Drawing for the job (mm, zero at the part's lowest x, y, z). A direction names the side the tool comes from. Round coordinates to 2 decimals unless told otherwise and drop trailing zeros. Write each loop counter-clockwise with the first axis right and the second up, starting at its lowest first coordinate (ties: lowest second). Pieces come first, ordered by that corner, then holes. Notation, with made-up numbers: M -38,-31.5 L -29,-31.5 A24 ccw -29,-6.5 Z; hole C 74,2.5 d4. An arc over 180 degrees is marked long. Use a Markdown table: item, result. Add a question column.
1) Slice it at D-D on x = 4.25. Write the cut outline in (y, z), plus the area to 3 significant figures.
2) Slice it at C-C on y = 3.75. Write the cut outline in (x, z).
3) Slice it at B-B on z = 4.25. Write the cut outline in (x, y).
4) Slice it at A-A on x = 7. Write the cut outline in (y, z).
5) Wall check: probe 1 along Y at (x, z) = (5, 4.75); probe 2 along X at (y, z) = (11.5, 4.5); probe 3 along Z at (x, y) = (6.25, 12.5). Give the ranges that are in metal, low to high.
6) Drop flat-ended pins along their axis: P1, Ø2, axis at y = 17, z = 5.5, coming from the +X side; P2, Ø8, axis at x = 6.5, y = 16.5, coming from the +Z side. Give the stop position or say it passes through.
7) Which spindle directions (+Z, -Z, +X, -X, +Y, -Y) get a long thin tool onto all of the face, cutting with end or side? Do the marked faces 1, 2 and 3. Say none if no direction does.
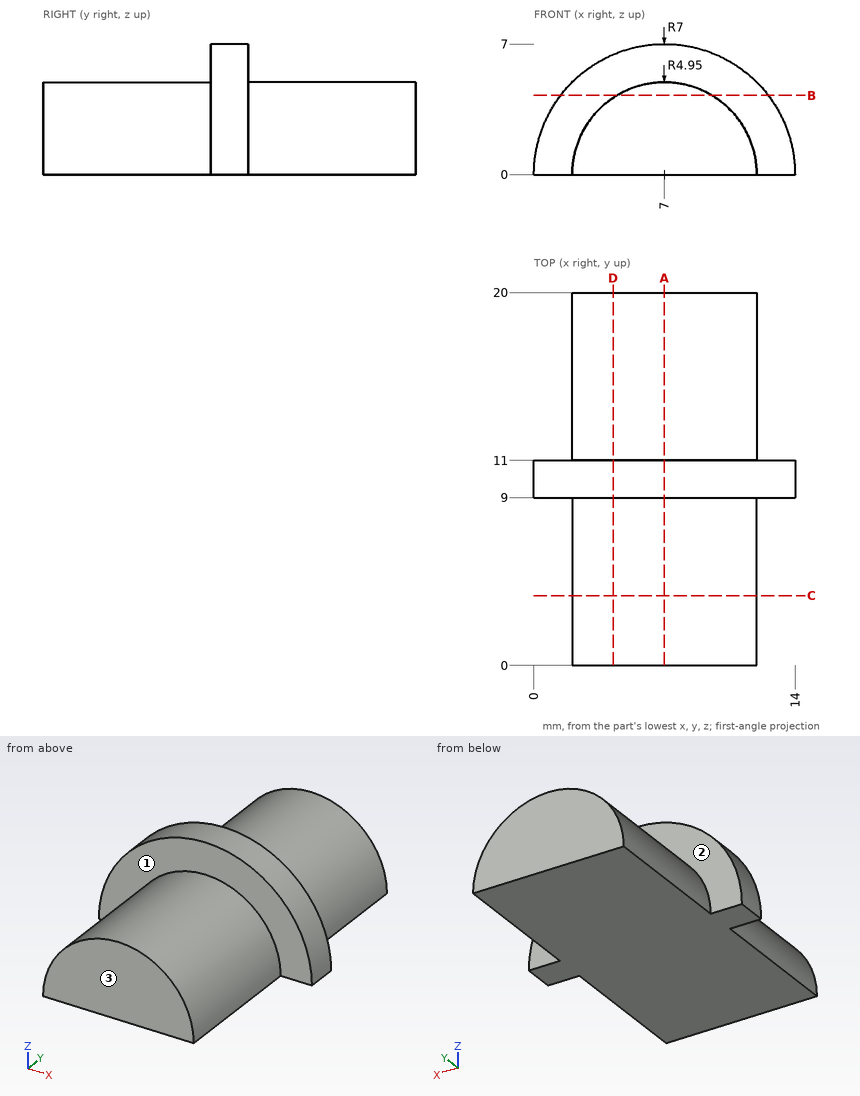
Entries:
| question | item | result |
|---|---|---|
| 1 | outline | M 0,0 L 20,0 L 20,4.12 L 11,4.12 L 11,6.44 L 9,6.44 L 9,4.12 L 0,4.12 Z |
| 1 | area | 87.0 mm^2 |
| 2 | outline | M 2.05,0 L 11.95,0 A4.95 ccw Z |
| 3 | outline | M 1.44,9 L 4.46,9 L 4.46,0 L 9.54,0 L 9.54,9 L 12.56,9 L 12.56,11 L 9.54,11 L 9.54,20 L 4.46,20 L 4.46,11 L 1.44,11 Z |
| 4 | outline | M 0,0 L 20,0 L 20,4.95 L 11,4.95 L 11,7 L 9,7 L 9,4.95 L 0,4.95 Z |
| 5 | probe 1 | y = 9 to 11 |
| 5 | probe 2 | x = 4.94 to 9.06 |
| 5 | probe 3 | z = 0 to 4.89 |
| 6 | P1 | stops at x = 9.06 |
| 6 | P2 | stops at z = 4.95 |
| 7 | face 1 | +Z, -Y |
| 7 | face 2 | +Z, +Y |
| 7 | face 3 | +Z, -Z, +X, -X, -Y |
